Source: CAD feature listing. Evaluate the final solid. Frame: model axes, mm. Face numbers are marked on the shaded views. A direction names the side the tool comes from. Round coordinates to 2 decimals unless told otherwise and drop trailing zeros. Order: outer loops, then holes, each group sorted by start corner. A loop starts at its lowest first (then second) coordinate and runs counter-clockwise, first axis right, second up.
```python
from build123d import *

# Parameters (mm, degrees)
SKETCH1_R           = 3.25
BOSS_EXTRUDE1_DEPTH = 22.686
SKETCH6_R           = 4.7
BOSS_EXTRUDE2_DEPTH = 8
FILLET1_R           = 0.75
BOSS_EXTRUDE3_DEPTH = 2


with BuildPart() as part:
    # Sketch1 → Boss-Extrude1 (new body)
    with BuildSketch(Plane(origin=(0, 0, 0), x_dir=(1, 0, 0), z_dir=(0, 1, 0))):
        Circle(SKETCH1_R)
    extrude(amount=BOSS_EXTRUDE1_DEPTH)

    # Sketch6 → Boss-Extrude2 (add)
    with BuildSketch(Plane(origin=(0, 22.686, 0), x_dir=(1, 0, 0), z_dir=(0, 1, 0))):
        Circle(SKETCH6_R)
    extrude(amount=BOSS_EXTRUDE2_DEPTH)

    # Fillet1
    fillet1_edges = [part.edges().sort_by_distance(p)[0] for p in [
        (-4.7, 30.686, 0),
    ]]
    fillet(fillet1_edges, radius=FILLET1_R)

    # Sketch7 → Boss-Extrude3 (add)
    with BuildSketch(Plane.XZ.offset(-22.686)):
        with BuildLine():
            Line((-1.016, 4.588871757), (-1.016, 6.620871757))
            Line((-1.016, 6.620871757), (1.016, 6.620871757))
            Line((1.016, 6.620871757), (1.016, 4.588871757))
            ThreePointArc((1.016, 4.588871757), (0, 4.7), (-1.016, 4.588871757))
        make_face()
        with BuildLine():
            Line((1.016, -6.620871757), (1.016, -4.588871757))
            ThreePointArc((1.016, -4.588871757), (0, -4.7), (-1.016, -4.588871757))
            Line((-1.016, -4.588871757), (-1.016, -6.620871757))
            Line((-1.016, -6.620871757), (1.016, -6.620871757))
        make_face()
    extrude(amount=-BOSS_EXTRUDE3_DEPTH)


solid = part.part
```
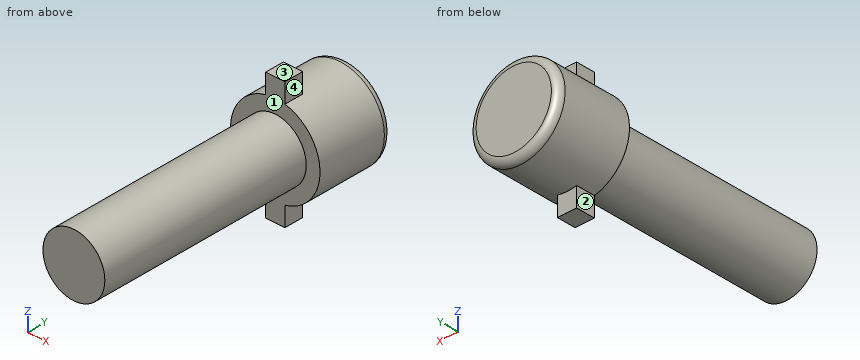
1. First-contact query: pin 1 (1.6 mm diameter, centred on y = 23.5, z = -5.5, fed in from -X); pin 2 (0.6 mm diameter, centred on x = -0.5, z = -6, fed in from +Y); pin 3 (1 mm diameter, centred on x = -2, y = 22, fed in from +Z); pin 4 (1.5 mm diameter, centred on y = 14.5, z = -4.5, fed in from -X). Flat tips, straight axial feed; report the tip coordinate or a pass-through.
2. Access query for the marked faces 1, 2, 3 and 4. Directions: +Z, -Z, +X, -X, +Y, -Y. A direction counts if a zero-diameter tool reaches every point of the face in a straight line with its end or side. Return the directions, or none.
3. Section D-D on z = 5.25. Return loops of the section in (x, y).
4. Line query: line 1 along Y through (x, z) = (-1.5, -3.5); line 2 along Z through (x, y) = (0, 12.5); line 3 along Z through (x, y) = (3.25, 26). Output: solid intervals per line, ascending.
5. Section A-A on z = 0. Return loops of the section in (x, y), plus the area to 3 significant figures.
6. Section C-C on y = 12.5. Return loops of the section in (x, z).
7. Section B-B on x = 0. Return loops of the section in (y, z).
Result:
1. pin 1: stops at x = -1.02
1. pin 2: stops at y = 24.69
1. pin 3: stops at z = 2.88
1. pin 4: passes through
2. face 1: -Y
2. face 2: -Z, -X, +Y, -Y
2. face 3: +Z, +X, -X, +Y, -Y
2. face 4: +Z, +X, +Y, -Y
3. outline: (-1.02, 22.69) - (1.02, 22.69) - (1.02, 24.69) - (-1.02, 24.69) - close
4. line 1: y = 22.69 to 30.69
4. line 2: z = -3.25 to 3.25
4. line 3: z = -3.4 to 3.4
5. outline: (-4.7, 22.69) - (-3.25, 22.69) - (-3.25, 0) - (3.25, 0) - (3.25, 22.69) - (4.7, 22.69) - (4.7, 29.94) arc R0.75 ccw to (3.95, 30.69) - (-3.95, 30.69) arc R0.75 ccw to (-4.7, 29.94) - close
5. area: 222 mm2
6. outline: circle Ø6.5 at (0, 0)
7. outline: (0, -3.25) - (22.69, -3.25) - (22.69, -6.62) - (24.69, -6.62) - (24.69, -4.7) - (29.94, -4.7) arc R0.75 ccw to (30.69, -3.95) - (30.69, 3.95) arc R0.75 ccw to (29.94, 4.7) - (24.69, 4.7) - (24.69, 6.62) - (22.69, 6.62) - (22.69, 3.25) - (0, 3.25) - close
